Can you work these out from the model? Positions are in its coordinate system, mm. A direction names the side the tool comes from. Give positions to 0.01 mm unless a question says otherwise; leave off trailing zeros. Loops run counter-clockwise (first coordinate to the right, second up) from the corner with the lowest first, then second, coordinate; pieces in that order, holes last. Notation, with made-up numbers: M -24,-19.75 L 32,-19.75 A7 ccw 32,-10.75 Z; hole C 63,1.25 d7. An arc over 180 degrees is marked long. Put each result on its own line as item: value. Start each with the question number.
1) For P1, Ø5, axis at y = 17.5, z = 7.5, coming from the +X side; P2, Ø2, axis at y = -24, z = 1, coming from the -X side; P3, Ø3.5, axis at x = 36, y = 16.5, coming from the +Z side, each with a flat end and sliding along its axis, tell me the tip position at first contact or that it passes through.
2) If we mould it in two halves opening along Y, with no side actions, what happens to faces 1 (the flat face through (-44, 19.7, 8.5)), 2 (the flat face through (-43.99, 10.71, 13.63)), 3 (the flat face through (-43, 24, 1))? For each: +Y half, -Y half, draft (parallel to the pull), parting line (faces both ways), or undercut.
3) Please list where these lines run through material, in increasing order: line 1 along Y through (x, z) = (-25, 1.5); line 2 along Z through (x, y) = (20, 3); line 3 along X through (y, z) = (-14.5, 2.25). Write a range as from..to.
4) Imagine slicing it at B-B (z = 15.75). Write out the boundary of the cut face in (x, y), then the cut area to 3 significant figures.
5) For faces 4 (the cylindrical face through (-25.202, 18.037, 1.014)), 5 (the flat face through (-45, 0, 7)), 6 (the flat face through (-44, 0, 12.67)), 7 (the flat face through (-43, 0, 8)), which set-ups out of +Z, -Z, +X, -X, +Y, -Y let a thin tool reach every point of the face, with its end or its side?
6) Imagine slicing it at A-A (x = -25). Write out the boundary of the cut face in (y, z).
7) Imagine slicing it at C-C (y = -6). Write out the boundary of the cut face in (x, z), then the cut area to 3 significant figures.
8) Imagine slicing it at D-D (x = 18). Write out the boundary of the cut face in (y, z), then the cut area to 3 significant figures.
from build123d import *

# Parameters (mm, degrees)
F0_W        = 86
F0_H        = 51
F1_DEPTH    = 2
F3_R        = 1.55
F4_DEPTH    = 25.4
F5_DEPTH    = 2
F6_T1_DEPTH = 9.0710678119


# Not quite as in the source:
# - a fillet or chamfer that OpenCascade refuses, or shapes differently, is made with other operations: its cross-section is extruded or revolved along the edge and cut away or added


with BuildPart() as f1:
    # F0 (on Top) → F1 (new body)
    with BuildSketch(Plane.XY):
        Rectangle(F0_W, F0_H)
    extrude(amount=F1_DEPTH)

    # F3 (on face) → F4 (cut)
    with BuildSketch(Plane.XY.offset(2)):
        with Locations((-25, 16.5)):
            Circle(F3_R)
        with Locations((-25, -16.5)):
            Circle(F3_R)
        with Locations((36, 16.5)):
            Circle(F3_R)
        with Locations((36, -16.5)):
            Circle(F3_R)
    extrude(amount=-F4_DEPTH, mode=Mode.SUBTRACT)

    # F2 (on face) → F5 (join)
    with BuildSketch(Plane(origin=(-43, 0, 0), x_dir=(0, -1, 0), z_dir=(-1, 0, 0))):
        with BuildLine():
            Line((8, 12.6704787835), (0, 12.6704787835))
            Line((0, 12.6704787835), (-8, 12.6704787835))
            Line((-8, 12.6704787835), (-13.5029918403, 14.6226324313))
            ThreePointArc((-13.5029918403, 14.6226324313), (-15.0300310094, 15.8378762171), (-15.4863987014, 17.7353468))
            Line((-15.4863987014, 17.7353468), (-16.9863987014, 17.7353468))
            Line((-16.9863987014, 17.7353468), (-16.9863987014, 16.7353468))
            Line((-16.9863987014, 16.7353468), (-22.5, 0))
            Line((-22.5, 0), (22.5, 0))
            Line((22.5, 0), (16.9863987014, 16.7353468))
            Line((16.9863987014, 16.7353468), (16.9863987014, 17.7353468))
            Line((16.9863987014, 17.7353468), (15.4863987014, 17.7353468))
            ThreePointArc((15.4863987014, 17.7353468), (15.0300310094, 15.8378762171), (13.5029918403, 14.6226324313))
            Line((13.5029918403, 14.6226324313), (8, 12.6704787835))
        make_face()
        with BuildLine():
            Line((8, 12.6704787835), (0, 12.6704787835))
            Line((0, 12.6704787835), (-8, 12.6704787835))
            Line((-8, 12.6704787835), (-13.5029918403, 14.6226324313))
            ThreePointArc((-13.5029918403, 14.6226324313), (-15.0300310094, 15.8378762171), (-15.4863987014, 17.7353468))
            Line((-15.4863987014, 17.7353468), (-16.9863987014, 17.7353468))
            Line((-16.9863987014, 17.7353468), (-16.9863987014, 16.7353468))
            Line((-16.9863987014, 16.7353468), (-21.8410831141, 2))
            Line((-21.8410831141, 2), (21.8410831141, 2))
            Line((21.8410831141, 2), (16.9863987014, 16.7353468))
            Line((16.9863987014, 16.7353468), (16.9863987014, 17.7353468))
            Line((16.9863987014, 17.7353468), (15.4863987014, 17.7353468))
            ThreePointArc((15.4863987014, 17.7353468), (15.0300310094, 15.8378762171), (13.5029918403, 14.6226324313))
            Line((13.5029918403, 14.6226324313), (8, 12.6704787835))
        make_face()
    extrude(amount=F5_DEPTH)

    # F6: fillet of radius 1.5 on 2 edges, made by hand

    # F6_s2 → F6_t1 (cut)
    with BuildSketch(Plane.YZ.offset(-48.5355339059)):
        with BuildLine():
            ThreePointArc((-15.572185139, 17.7353468), (-16.4382105428, 17.4600916714), (-16.9863987014, 16.7353468))
            Line((-16.9863987014, 16.7353468), (-16.9863987014, 17.7353468))
            Line((-16.9863987014, 17.7353468), (-15.572185139, 17.7353468))
        make_face()
        with BuildLine():
            ThreePointArc((16.9863987014, 16.7353468), (16.4382105428, 17.4600916714), (15.572185139, 17.7353468))
            Line((15.572185139, 17.7353468), (16.9863987014, 17.7353468))
            Line((16.9863987014, 17.7353468), (16.9863987014, 16.7353468))
        make_face()
    extrude(amount=F6_T1_DEPTH, mode=Mode.SUBTRACT)


solid = f1.part
Recorded:
1. P1: x = -43
1. P2: x = -43
1. P3: z = 2
2. face 1: +Y half
2. face 2: undercut
2. face 3: draft
3. line 1: -25.5..-18.05, -14.95..14.95, 18.05..25.5
3. line 2: 0..2
3. line 3: -45..-43
4. outline: M -45,-17.31 L -43,-17.31 L -43,-14.97 L -45,-14.97 Z; M -45,14.97 L -43,14.97 L -43,17.31 L -45,17.31 Z
4. area: 9.36 mm²
5. face 4: +Z, -Z
5. face 5: +Z, -Z, -X, +Y, -Y
5. face 6: +Z, +X, -X
5. face 7: +Z, +X, +Y, -Y
6. outline: M -25.5,0 L -18.05,0 L -18.05,2 L -25.5,2 Z; M -14.95,0 L 14.95,0 L 14.95,2 L -14.95,2 Z; M 18.05,0 L 25.5,0 L 25.5,2 L 18.05,2 Z
7. outline: M -45,0 L 43,0 L 43,2 L -43,2 L -43,12.67 L -45,12.67 Z
7. area: 197 mm²
8. outline: M -25.5,0 L 25.5,0 L 25.5,2 L -25.5,2 Z
8. area: 102 mm²
